```python
from build123d import *

# Parameters (mm, degrees)
SKETCH1_R           = 3.175
BOSS_EXTRUDE1_DEPTH = 3.81
BOSS_EXTRUDE2_START = 4.7625
SKETCH4_R           = 9.525
SKETCH4_R_2         = 6.985
SKETCH4_R_3         = 3.175
BOSS_EXTRUDE2_DEPTH = 4.7625
BOSS_EXTRUDE3_START = -0.79375
BOSS_EXTRUDE3_DEPTH = 3.175
CIRPATTERN1_COUNT   = 5
SKETCH6_R           = 1.5875
SKETCH7_R           = 1.675
CUT_EXTRUDE1_DEPTH  = 16.96680952


with BuildPart() as part:
    # Sketch1 → Boss-Extrude1 (new body)
    with BuildSketch(Plane(origin=(0, 0, 0), x_dir=(0, 0, -1), z_dir=(1, 0, 0))):
        with Locations(Location((0, 0, 0), (0, 0, 180))):
            Circle(SKETCH1_R)
    extrude(amount=BOSS_EXTRUDE1_DEPTH)

    # Sketch4 → Boss-Extrude2 (add)
    # profile 1 of 2: a face of its own
    with BuildSketch(Plane.ZY.offset(BOSS_EXTRUDE2_START)):
        with Locations(Location((0, 0, 0), (0, 0, 180))):
            Circle(SKETCH4_R)
        with Locations(Location((0, 0, 0), (0, 0, 180))):
            Circle(SKETCH4_R_2, mode=Mode.SUBTRACT)
    # profile 2 of 2: a face of its own
    with BuildSketch(Plane.ZY.offset(BOSS_EXTRUDE2_START)):
        Circle(SKETCH4_R_3)
    extrude(amount=-BOSS_EXTRUDE2_DEPTH)


with BuildPart() as boss_extrude2_piece_1:
    # of the separate pieces the step leaves, piece 1, a body of its own (boss_extrude2_pieces)
    add(part.part.solids().sort_by_distance((-4.7625, 0, -9.525))[0])



with BuildPart() as boss_extrude2_piece_2:
    # of the separate pieces the step leaves, piece 2, a body of its own (boss_extrude2_pieces)
    add(part.part.solids().sort_by_distance((3.81, 0, 3.175))[0])


with BuildPart() as boss_extrude2_piece_1_1:
    add(boss_extrude2_piece_1.part)

    add(boss_extrude2_piece_2.part)  # Boss-Extrude3 merges Boss-Extrude2 piece 2
    # Sketch5 → Boss-Extrude3 (add)
    with BuildSketch(Plane.ZY.offset(4.7625).offset(BOSS_EXTRUDE3_START)):
        with BuildLine():
            Line((0, 0), (1.212932521, 6.878882155))
            ThreePointArc((1.212932521, 6.878882155), (0, 6.985), (-1.212932521, 6.878882155))
            Line((-1.212932521, 6.878882155), (0, 0))
        make_face()
    boss_extrude3 = extrude(amount=-BOSS_EXTRUDE3_DEPTH)

    # CirPattern1: Boss-Extrude3 ×5 about axis
    cirpattern1_axis = Axis((0, 0, 0), (1, 0, 0))
    for i in range(1, CIRPATTERN1_COUNT):
        add(boss_extrude3.rotate(cirpattern1_axis, i * 360 / CIRPATTERN1_COUNT))

    # Sketch6 → Cut-Revolve1 (revolve, cut)
    with BuildSketch(Plane(origin=(0, 0, 0), x_dir=(1, 0, 0), z_dir=(0, 1, 0))):
        with Locations((-2.38125, 9.525)):
            Circle(SKETCH6_R)
    revolve(axis=Axis((3.81, 0, 0), (-1, 0, 0)), mode=Mode.SUBTRACT)

    # Sketch7 → Cut-Extrude1 (cut, through all)
    with BuildSketch(Plane.ZY.offset(4.7625)):
        Circle(SKETCH7_R)
    extrude(amount=-CUT_EXTRUDE1_DEPTH, mode=Mode.SUBTRACT)


solid = boss_extrude2_piece_1_1.part
```
Build history of the part. All positions in model axes, mm. A direction names the side the tool comes from. Give positions to 0.01 mm unless a question says otherwise; leave off trailing zeros. Loops run counter-clockwise (first coordinate to the right, second up) from the corner with the lowest first, then second, coordinate; pieces in that order, holes last. Notation, with made-up numbers: (-36.75, -7) -> (2.25, -7) arc R27 cw to (2.25, 32) -> close; hole circle Ø9 at (41, 55.25). An arc over 180 degrees is marked (long way). One line per question, with ' | ' between items.
Q1. Cut at C-C, the plane x = -3.25. Write the cut outline in (y, z) (3 decimals).
Filled sheet:
outline: circle Ø16.393 at (0, 0); hole (-6.278, -3.062) -> (-2.854, -1.392) arc R3.175 cw to (-2.854, 1.392) -> (-6.278, 3.062) arc R6.985 ccw to start; hole (-4.852, -5.025) arc R6.985 ccw to (0.972, -6.917) -> (0.442, -3.144) arc R3.175 cw to (-2.206, -2.284) -> close; hole (-4.852, 5.025) -> (-2.206, 2.284) arc R3.175 cw to (0.442, 3.144) -> (0.972, 6.917) arc R6.985 ccw to start; hole circle Ø3.35 at (0, 0); hole (1.491, -2.803) -> (3.279, -6.167) arc R6.985 ccw to (6.879, -1.213) -> (3.127, -0.551) arc R3.175 cw to start; hole (1.491, 2.803) arc R3.175 cw to (3.127, 0.551) -> (6.879, 1.213) arc R6.985 ccw to (3.279, 6.167) -> close
Q2. Tool access for faces 5 (the flat face through (-3.969, -4, -3)), 6 (the flat face through (-2.4, 0.71, -5.06)), 7 (the flat face through (-0.794, 6, 0)): list every direction of +Z, -Z, +X, -X, +Y, -Y with a clear straight run to the whole face (end or side of a thin tool).
Filled sheet:
face 5: -X | face 6: +X, -X | face 7: +X
Q3. Pull direction Z, two halves, no side cores. Call faces 1 (the cylindrical face through (-0.536, 0.074, -1.673)), 2 (the flat face through (-4.762, -1.4, 1.4)), 3 (the cylindrical face through (-4.37, 9.3, 2.06)), 4 (the flat face through (-0.794, 2, 5)): pulls with the +Z half, pulls with the -Z half, needs draft (parallel to the pull), parting line crosses it, or undercut.
Filled sheet:
face 1: undercut | face 2: needs draft | face 3: parting line crosses it | face 4: undercut
Q4. Drill centre lines: line 1 along Y through (x, z) = (-2.5, 0) (3 decimals); line 2 along Y through (x, z) = (2.25, 0) (3 decimals); line 3 along Y through (x, z) = (-3.15, 0) (3 decimals). Where is each one in solid material? Low to high. Write a range as [from, to].
Filled sheet:
line 1: y = [-7.942, -6.985], [-3.175, -1.675], [1.675, 7.942] | line 2: y = [-3.175, -1.675], [1.675, 3.175] | line 3: y = [-8.136, -6.985], [-3.175, -1.675], [1.675, 8.136]
Q5. Cut at D-D, the plane x = 2. Write the cut outline in (y, z) (3 decimals), plus the area to 3 significant figures.
Filled sheet:
outline: circle Ø6.35 at (0, 0); hole circle Ø3.35 at (0, 0) | area: 22.9 mm²
Q6. Cut at B-B, the plane z = 0. Write the cut outline in (x, y) (1 decimal), plus the area to 3 significant figures.
Filled sheet:
outline: (-4.8, -9.5) -> (-4, -9.5) arc R1.6 cw to (-0.8, -9.5) -> (0, -9.5) -> (0, -7) -> (-4.8, -7) -> close; (-4.8, -3.2) -> (3.8, -3.2) -> (3.8, -1.7) -> (-4.8, -1.7) -> close; (-4.8, 1.7) -> (3.8, 1.7) -> (3.8, 3.2) -> (-0.8, 3.2) -> (-0.8, 7) -> (0, 7) -> (0, 9.5) -> (-0.8, 9.5) arc R1.6 cw to (-4, 9.5) -> (-4.8, 9.5) -> (-4.8, 7) -> (-4, 7) -> (-4, 3.2) -> (-4.8, 3.2) -> close | area: 54.1 mm²
Q7. Drop flat-ended pins along their axis: pin 1 (0.7 mm diameter, centred on y = 4, z = 0, fed in from +X); pin 2 (2.5 mm diameter, centred on y = 5, z = -0.5, fed in from -X); pin 3 (5 mm diameter, centred on x = -2, y = 4.5, fed in from +Z). Give the stop position or say it passes through.
Filled sheet:
pin 1: stops at x = -0.79 | pin 2: stops at x = -3.97 | pin 3: stops at z = 9.24
Q8. Cut at A-A, the plane y = 0. Write the cut outline in (x, z) (1 decimal).
Filled sheet:
outline: (-4.8, -9.5) -> (-4, -9.5) arc R1.6 cw to (-0.8, -9.5) -> (0, -9.5) -> (0, -7) -> (-4.8, -7) -> close; (-4.8, -3.2) -> (3.8, -3.2) -> (3.8, -1.7) -> (-4.8, -1.7) -> close; (-4.8, 1.7) -> (3.8, 1.7) -> (3.8, 3.2) -> (-4.8, 3.2) -> close; (-4.8, 7) -> (0, 7) -> (0, 9.5) -> (-0.8, 9.5) arc R1.6 cw to (-4, 9.5) -> (-4.8, 9.5) -> close
